from build123d import *

# Parameters (mm, degrees)
F0_W           = 52
F0_H           = 67.66
F2_DEPTH       = 5
F1_R           = 3.265
F3_DEPTH       = 5
F4_W           = 52
F4_H           = 67.66
F5_DEPTH       = 30
F7_W           = 52
F7_H           = 67.66
F8_DEPTH       = 25
F9_W           = 100
F9_H           = 100
F10_DEPTH      = 10
F12_DEPTH      = 10
F6_W           = 17.5
F6_H           = 17.5
F6_W_2         = 25
F13_DEPTH      = 30
F13_DEPTH_BACK = 10


with BuildPart() as f2:
    # F0 (on Top) → F2 (new body)
    with BuildSketch(Plane.XY):
        with Locations((0, -3.83)):
            Rectangle(F0_W, F0_H)
    extrude(amount=F2_DEPTH)

    # F1 (on face) → F3 (cut)
    with BuildSketch(Plane.XY):
        with Locations((-18, 20)):
            Circle(F1_R)
        with Locations((18, 20)):
            Circle(F1_R)
        with Locations((0, -28)):
            Circle(F1_R)
    extrude(amount=F3_DEPTH, mode=Mode.SUBTRACT)

    # F4 (on face) → F5 (join)
    with BuildSketch(Plane.XY.offset(5)):
        with Locations((0, -3.83)):
            Rectangle(F4_W, F4_H)
    extrude(amount=F5_DEPTH)

    # F7 (on face) → F8 (join)
    with BuildSketch(Plane.XY.offset(35)):
        with Locations((0, -3.83)):
            Rectangle(F7_W, F7_H)
    extrude(amount=F8_DEPTH)

    # F9 (on face) → F10 (join)
    with BuildSketch(Plane.XY.offset(60)):
        Rectangle(F9_W, F9_H)
    extrude(amount=-F10_DEPTH)

    # F11 (on face) → F12 (cut)
    with BuildSketch(Plane.XY.offset(60)):
        with BuildLine():
            Line((34.835, -6.35), (41.365, -6.35))
            ThreePointArc((41.365, -6.35), (38.1, -3.085), (34.835, -6.35))
        make_face()
        with BuildLine():
            ThreePointArc((34.835, -6.35), (38.1, -9.615), (41.365, -6.35))
            Line((41.365, -6.35), (34.835, -6.35))
        make_face()
        with BuildLine():
            ThreePointArc((34.835, -6.35), (38.1, -3.085), (41.365, -6.35))
            Line((41.365, -6.35), (41.365, 6.35))
            ThreePointArc((41.365, 6.35), (38.1, 3.085), (34.835, 6.35))
            Line((34.835, 6.35), (34.835, -6.35))
        make_face()
        with BuildLine():
            Line((34.835, 6.35), (41.365, 6.35))
            ThreePointArc((41.365, 6.35), (38.1, 9.615), (34.835, 6.35))
        make_face()
        with BuildLine():
            ThreePointArc((34.835, 6.35), (38.1, 3.085), (41.365, 6.35))
            Line((41.365, 6.35), (34.835, 6.35))
        make_face()
        with BuildLine():
            Line((34.835, -31.75), (41.365, -31.75))
            ThreePointArc((41.365, -31.75), (38.1, -28.485), (34.835, -31.75))
        make_face()
        with BuildLine():
            ThreePointArc((34.835, -31.75), (38.1, -35.015), (41.365, -31.75))
            Line((41.365, -31.75), (34.835, -31.75))
        make_face()
        with BuildLine():
            ThreePointArc((34.835, -31.75), (38.1, -28.485), (41.365, -31.75))
            Line((41.365, -31.75), (41.365, -19.05))
            ThreePointArc((41.365, -19.05), (38.1, -22.315), (34.835, -19.05))
            Line((34.835, -19.05), (34.835, -31.75))
        make_face()
        with BuildLine():
            Line((34.835, -19.05), (41.365, -19.05))
            ThreePointArc((41.365, -19.05), (38.1, -15.785), (34.835, -19.05))
        make_face()
        with BuildLine():
            ThreePointArc((34.835, -19.05), (38.1, -22.315), (41.365, -19.05))
            Line((41.365, -19.05), (34.835, -19.05))
        make_face()
        with BuildLine():
            ThreePointArc((34.835, 31.75), (38.1, 28.485), (41.365, 31.75))
            ThreePointArc((41.365, 31.75), (38.1, 35.015), (34.835, 31.75))
        make_face()
        with BuildLine():
            Line((41.365, 19.05), (41.365, 31.75))
            ThreePointArc((41.365, 31.75), (38.1, 28.485), (34.835, 31.75))
            Line((34.835, 31.75), (34.835, 19.05))
            ThreePointArc((34.835, 19.05), (38.1, 22.315), (41.365, 19.05))
        make_face()
        with BuildLine():
            ThreePointArc((34.835, 19.05), (38.1, 15.785), (41.365, 19.05))
            ThreePointArc((41.365, 19.05), (38.1, 22.315), (34.835, 19.05))
        make_face()
        with BuildLine():
            ThreePointArc((-41.365, -31.75), (-38.1, -35.015), (-34.835, -31.75))
            ThreePointArc((-34.835, -31.75), (-38.1, -28.485), (-41.365, -31.75))
        make_face()
        with BuildLine():
            ThreePointArc((-41.365, -31.75), (-38.1, -28.485), (-34.835, -31.75))
            Line((-34.835, -31.75), (-34.835, -19.05))
            ThreePointArc((-34.835, -19.05), (-38.1, -22.315), (-41.365, -19.05))
            Line((-41.365, -19.05), (-41.365, -31.75))
        make_face()
        with BuildLine():
            ThreePointArc((-41.365, -19.05), (-38.1, -22.315), (-34.835, -19.05))
            ThreePointArc((-34.835, -19.05), (-38.1, -15.785), (-41.365, -19.05))
        make_face()
        with BuildLine():
            ThreePointArc((-41.365, -6.35), (-38.1, -9.615), (-34.835, -6.35))
            ThreePointArc((-34.835, -6.35), (-38.1, -3.085), (-41.365, -6.35))
        make_face()
        with BuildLine():
            ThreePointArc((-41.365, -6.35), (-38.1, -3.085), (-34.835, -6.35))
            Line((-34.835, -6.35), (-34.835, 6.35))
            ThreePointArc((-34.835, 6.35), (-38.1, 3.085), (-41.365, 6.35))
            Line((-41.365, 6.35), (-41.365, -6.35))
        make_face()
        with BuildLine():
            ThreePointArc((-41.365, 6.35), (-38.1, 3.085), (-34.835, 6.35))
            ThreePointArc((-34.835, 6.35), (-38.1, 9.615), (-41.365, 6.35))
        make_face()
        with BuildLine():
            ThreePointArc((-41.365, 19.05), (-38.1, 15.785), (-34.835, 19.05))
            ThreePointArc((-34.835, 19.05), (-38.1, 22.315), (-41.365, 19.05))
        make_face()
        with BuildLine():
            ThreePointArc((-41.365, 19.05), (-38.1, 22.315), (-34.835, 19.05))
            Line((-34.835, 19.05), (-34.835, 31.75))
            ThreePointArc((-34.835, 31.75), (-38.1, 28.485), (-41.365, 31.75))
            Line((-41.365, 31.75), (-41.365, 19.05))
        make_face()
        with BuildLine():
            ThreePointArc((-41.365, 31.75), (-38.1, 28.485), (-34.835, 31.75))
            ThreePointArc((-34.835, 31.75), (-38.1, 35.015), (-41.365, 31.75))
        make_face()
    extrude(amount=-F12_DEPTH, mode=Mode.SUBTRACT)

    # F6 (on face) → F13 (cut, two sides)
    with BuildSketch(Plane.XY.offset(35)) as f13_sk:
        with Locations((-17.25, 21.25)):
            Rectangle(F6_W, F6_H)
        with Locations((17.25, 21.25)):
            Rectangle(F6_W, F6_H)
        with Locations((0, -28.91)):
            Rectangle(F6_W_2, F6_H)
    extrude(amount=-F13_DEPTH, mode=Mode.SUBTRACT)
    extrude(f13_sk.sketch, amount=F13_DEPTH_BACK, mode=Mode.SUBTRACT)


solid = f2.part
The listing builds one solid part. Answer for the finished solid, in the listing's coordinates (mm). A direction names the side the tool comes from. Give positions to 0.01 mm unless a question says otherwise; leave off trailing zeros. Loops run counter-clockwise (first coordinate to the right, second up) from the corner with the lowest first, then second, coordinate; pieces in that order, holes last. Notation, with made-up numbers: (-31.5, 23.5) - (-4.5, 23.5) arc R28 cw to (-4.5, 56.5) - close; hole circle Ø5 at (89.25, 20). An arc over 180 degrees is marked (long way). Write each question's results on one line, items separated by ' | '.
1. Flat-ended cylindrical pins translate along their axes: P1, Ø5, axis at x = 37, y = 21, coming from the +Z side; P2, Ø19, axis at y = -28, z = 32, coming from the -X side; P3, Ø6, axis at x = -15, z = 7.5, coming from the +Y side; P4, Ø2, axis at x = -34.5, y = 7, coming from the -Z side. Find the tip coordinate at first contact, or state that the pin passes through.
Resolved:
P1: stops at z = 60 | P2: stops at x = -26 | P3: stops at y = 30 | P4: stops at z = 50
2. For a pull along Z with two mould halves and no side action, classify faces 5 (the face through (21.114, 20.981, 2.465)), 6 (the face through (-8.5, 21, 25)) as +Z half, -Z half, draft (parallel to the pull), parting line (faces both ways), or undercut.
Resolved:
face 5: draft | face 6: undercut
3. Find section B-B, the plane y = 3. Write down the section's boundary in (x, z) (3 decimals).
Resolved:
outline: (-50, 50) - (-41.365, 50) - (-41.365, 60) - (-50, 60) - close; (-34.835, 50) - (-26, 50) - (-26, 0) - (26, 0) - (26, 50) - (34.835, 50) - (34.835, 60) - (-34.835, 60) - close; (41.365, 50) - (50, 50) - (50, 60) - (41.365, 60) - close
4. Find section C-C, the plane z = 55.5. Write down the section's boundary in (x, y) (3 decimals).
Resolved:
outline: (-50, -50) - (50, -50) - (50, 50) - (-50, 50) - close; hole (-41.365, -31.75) arc R3.265 ccw to (-34.835, -31.75) - (-34.835, -19.05) arc R3.265 ccw to (-41.365, -19.05) - close; hole (-41.365, -6.35) arc R3.265 ccw to (-34.835, -6.35) - (-34.835, 6.35) arc R3.265 ccw to (-41.365, 6.35) - close; hole (-41.365, 19.05) arc R3.265 ccw to (-34.835, 19.05) - (-34.835, 31.75) arc R3.265 ccw to (-41.365, 31.75) - close; hole (34.835, -31.75) arc R3.265 ccw to (41.365, -31.75) - (41.365, -19.05) arc R3.265 ccw to (34.835, -19.05) - close; hole (34.835, -6.35) arc R3.265 ccw to (41.365, -6.35) - (41.365, 6.35) arc R3.265 ccw to (34.835, 6.35) - close; hole (34.835, 19.05) arc R3.265 ccw to (41.365, 19.05) - (41.365, 31.75) arc R3.265 ccw to (34.835, 31.75) - close
5. Find section A-A, the plane x = -38.1. Write down the section's boundary in (y, z) (3 decimals).
Resolved:
outline: (-50, 50) - (-35.015, 50) - (-35.015, 60) - (-50, 60) - close; (-15.785, 50) - (-9.615, 50) - (-9.615, 60) - (-15.785, 60) - close; (9.615, 50) - (15.785, 50) - (15.785, 60) - (9.615, 60) - close; (35.015, 50) - (50, 50) - (50, 60) - (35.015, 60) - close
6. Find section D-D, the plane x = -7. Write down the section's boundary in (y, z).
Resolved:
outline: (-50, 50) - (-37.66, 50) - (-37.66, 45) - (-20.16, 45) - (-20.16, 5) - (-37.66, 5) - (-37.66, 0) - (30, 0) - (30, 50) - (50, 50) - (50, 60) - (-50, 60) - close
7. Which of the six approach directions +Z, -Z, +X, -X, +Y, -Y give full straight-line access (tool end or side, diameter ignored) to faces 1 (the face through (-38.028, -15.786, 55.07)), 2 (the face through (-14.886, 20.981, 2.465)), 3 (the face through (-15, 23, 5)), 4 (the face through (-26, -12, 25))?
Resolved:
face 1: +Z, -Z | face 2: -Z | face 3: -X, +Y | face 4: -Z, -X, +Y, -Y
8. Consider probe 1 along X at (y, z) = (25, 51) (3 decimals); probe 2 along Y at (x, z) = (0, 1.75) (3 decimals); probe 3 along Y at (x, z) = (18, 3) (3 decimals). Determine where each line is inside the solid, lowest interval first. Write a range as from..to.
Resolved:
probe 1: x = -50..-41.365, -34.835..34.835, 41.365..50 | probe 2: y = -37.66..-31.265, -24.735..30 | probe 3: y = -37.66..16.735, 23.265..30
